```python
from build123d import *

# Parameters (mm, degrees)
SKETCH_1_R          = 40
EXTRUDE_1_DEPTH     = 11.8
SKETCH_2_R          = 2.15
SKETCH_2_R_2        = 1.75
CUT_EXTRUDE_1_DEPTH = 58.786157512
SKETCH_3_R          = 3.925
SKETCH_3_R_2        = 15.6
CUT_EXTRUDE_2_DEPTH = 58.786157512
SKETCH_5_R          = 2.9
SKETCH_5_R_2        = 3.5
CUT_EXTRUDE_4_DEPTH = 4
CHAMFER_1_SIZE      = 0.5


with BuildPart() as part:
    # 草图1 → 凸台-拉伸1 (new body)
    with BuildSketch(Plane.XY):
        Circle(SKETCH_1_R)
    extrude(amount=EXTRUDE_1_DEPTH)

    # 草图2 → 切除-拉伸1 (cut, through all)
    with BuildSketch(Plane(origin=(0, 0, 0), x_dir=(-1, 0, 0), z_dir=(0, 0, -1))):
        with Locations((-32.730643847, 10.1245665)):
            Circle(SKETCH_2_R)
        with Locations(Location((-32.730643847, -9.8754335, 0), (0, 0, 180))):
            Circle(SKETCH_2_R)
        with Locations((32.269356153, -9.8754335)):
            Circle(SKETCH_2_R)
        with Locations(Location((32.269356153, 10.1245665, 0), (0, 0, 180))):
            Circle(SKETCH_2_R)
        with Locations((-9.290643847, 33.9345665)):
            Circle(SKETCH_2_R_2)
        with Locations(Location((8.829356153, 33.9345665, 0), (0, 0, 180))):
            Circle(SKETCH_2_R_2)
        with Locations((8.829356153, -33.6854335)):
            Circle(SKETCH_2_R_2)
        with Locations(Location((-9.290643847, -33.6854335, 0), (0, 0, 180))):
            Circle(SKETCH_2_R_2)
    extrude(amount=-CUT_EXTRUDE_1_DEPTH, mode=Mode.SUBTRACT)

    # 草图3 → 切除-拉伸2 (cut, through all)
    with BuildSketch(Plane(origin=(0, 0, 0), x_dir=(-1, 0, 0), z_dir=(0, 0, -1))):
        with Locations((0, 31.5)):
            Circle(SKETCH_3_R)
        with Locations((27.279800219, 15.75)):
            Circle(SKETCH_3_R)
        with Locations((27.279800219, -15.75)):
            Circle(SKETCH_3_R)
        with Locations((0, -31.5)):
            Circle(SKETCH_3_R)
        with Locations((-27.279800219, -15.75)):
            Circle(SKETCH_3_R)
        with Locations((-27.279800219, 15.75)):
            Circle(SKETCH_3_R)
        Circle(SKETCH_3_R_2)
    extrude(amount=-CUT_EXTRUDE_2_DEPTH, mode=Mode.SUBTRACT)

    # 草图5 → 切除-拉伸4 (cut)
    with BuildSketch(Plane.XY.offset(11.8)):
        with Locations((-8.829356153, -33.6854335)):
            Circle(SKETCH_5_R)
        with Locations((-8.829356153, 33.9345665)):
            Circle(SKETCH_5_R)
        with Locations((-32.269356153, 10.1245665)):
            Circle(SKETCH_5_R_2)
        with Locations((-32.269356153, -9.8754335)):
            Circle(SKETCH_5_R_2)
        with Locations((9.290643847, 33.9345665)):
            Circle(SKETCH_5_R)
        with Locations((32.730643847, 10.1245665)):
            Circle(SKETCH_5_R_2)
        with Locations((32.730643847, -9.8754335)):
            Circle(SKETCH_5_R_2)
        with Locations((9.290643847, -33.6854335)):
            Circle(SKETCH_5_R)
    extrude(amount=-CUT_EXTRUDE_4_DEPTH, mode=Mode.SUBTRACT)

    # 倒角1
    # the kernel refuses this chamfer: 0.5 mm, written as the material it takes off along each edge
    with BuildSketch(Plane(origin=(0, 31.5, 11.8), x_dir=(-1, 0, 0), z_dir=(0, -1, 0))) as chamfer_1_piece_1:
        Polygon((3.925 + CHAMFER_1_SIZE, 0), (3.925, CHAMFER_1_SIZE), (3.925, 0), align=None)
    revolve(axis=Axis((0, 31.5, 11.8), (0, 0, -1)), mode=Mode.SUBTRACT)
    with BuildSketch(Plane(origin=(0, -31.5, 11.8), x_dir=(-1, 0, 0), z_dir=(0, -1, 0))) as chamfer_1_piece_2:
        Polygon((3.925 + CHAMFER_1_SIZE, 0), (3.925, CHAMFER_1_SIZE), (3.925, 0), align=None)
    revolve(axis=Axis((0, -31.5, 11.8), (0, 0, -1)), mode=Mode.SUBTRACT)
    with BuildSketch(Plane(origin=(-27.279800219, -15.75, 11.8), x_dir=(-1, 0, 0), z_dir=(0, -1, 0))) as chamfer_1_piece_3:
        Polygon((3.925 + CHAMFER_1_SIZE, 0), (3.925, CHAMFER_1_SIZE), (3.925, 0), align=None)
    revolve(axis=Axis((-27.279800219, -15.75, 11.8), (0, 0, -1)), mode=Mode.SUBTRACT)
    with BuildSketch(Plane(origin=(-27.279800219, 15.75, 11.8), x_dir=(-1, 0, 0), z_dir=(0, -1, 0))) as chamfer_1_piece_4:
        Polygon((3.925 + CHAMFER_1_SIZE, 0), (3.925, CHAMFER_1_SIZE), (3.925, 0), align=None)
    revolve(axis=Axis((-27.279800219, 15.75, 11.8), (0, 0, -1)), mode=Mode.SUBTRACT)
    with BuildSketch(Plane(origin=(27.279800219, -15.75, 11.8), x_dir=(-1, 0, 0), z_dir=(0, -1, 0))) as chamfer_1_piece_5:
        Polygon((3.925 + CHAMFER_1_SIZE, 0), (3.925, CHAMFER_1_SIZE), (3.925, 0), align=None)
    revolve(axis=Axis((27.279800219, -15.75, 11.8), (0, 0, -1)), mode=Mode.SUBTRACT)
    with BuildSketch(Plane(origin=(27.279800219, 15.75, 11.8), x_dir=(-1, 0, 0), z_dir=(0, -1, 0))) as chamfer_1_piece_6:
        Polygon((3.925 + CHAMFER_1_SIZE, 0), (3.925, CHAMFER_1_SIZE), (3.925, 0), align=None)
    revolve(axis=Axis((27.279800219, 15.75, 11.8), (0, 0, -1)), mode=Mode.SUBTRACT)


solid = part.part
```
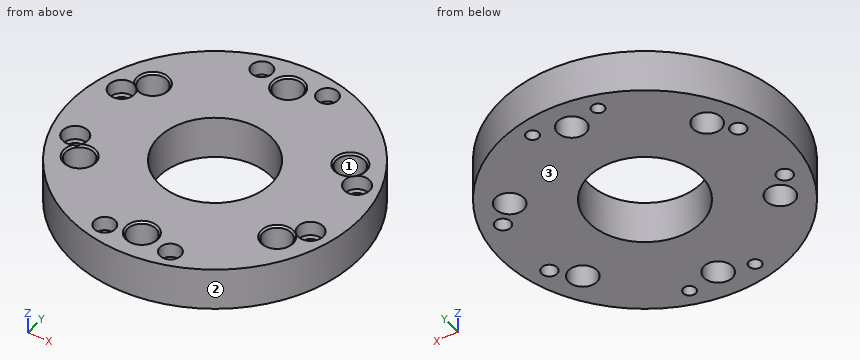
Work out the finished part from the listing and answer in its coordinate system (mm). Face numbers are marked on the shaded views. Give positions to 0.01 mm unless a question says otherwise; leave off trailing zeros. Loops run counter-clockwise (first coordinate to the right, second up) from the corner with the lowest first, then second, coordinate; pieces in that order, holes last. Notation, with made-up numbers: (0, 22) - (9, 22) arc R10 cw to (9, 41) - close; hole circle Ø3 at (-8.5, 73.5). An arc over 180 degrees is marked (long way). One line per question, with ' | ' between items.
(1) Each of these flat-tipped pins is pushed along its axis until it touches: pin 1 Ø1.5 at (y, z) = (8, 8.5) entering from -X; pin 2 Ø5 at (x, z) = (11.5, 2.5) entering from -Y; pin 3 Ø7 at (x, y) = (27.28, 15.75) entering from +Z; pin 4 Ø1.5 at (y, z) = (21.5, 9.5) entering from +X. Where does it stop, or does it pass through?
Recorded:
pin 1: stops at x = -39.34 | pin 2: stops at y = -38.97 | pin 3: passes through | pin 4: stops at x = 34.2
(2) The part is cut by section D-D (x = -13.5). Write down the section's boundary in (y, z), then the cut area to 3 significant figures.
Recorded:
outline: (-37.65, 0) - (-7.82, 0) - (-7.82, 11.8) - (-37.65, 11.8) - close; (7.82, 0) - (37.65, 0) - (37.65, 11.8) - (7.82, 11.8) - close | area: 704 mm²
(3) The part is cut by section C-C (z = 8.75). Count the separate pieces of the cut face and the enclosed holes in it, then the cut area to 3 significant figures.
Recorded:
separate pieces: 1 | enclosed holes: 15 | area: 3,710 mm²
(4) The part is cut by section B-B (x = 0). Write down the section's boundary in (y, z) (3 decimals), then the cut area to 3 significant figures.
Recorded:
outline: (-40, 0) - (-35.425, 0) - (-35.425, 11.3) - (-35.925, 11.8) - (-40, 11.8) - close; (-27.575, 0) - (-15.6, 0) - (-15.6, 11.8) - (-27.075, 11.8) - (-27.575, 11.3) - close; (15.6, 0) - (27.575, 0) - (27.575, 11.3) - (27.075, 11.8) - (15.6, 11.8) - close; (35.425, 0) - (40, 0) - (40, 11.8) - (35.925, 11.8) - (35.425, 11.3) - close | area: 390 mm²
(5) The mould has two halves that part along Y. Classify the marked faces 1, 2 and 3: +Y half, -Y half, draft (parallel to the pull), parting line (faces both ways), or undercut.
Recorded:
face 1: undercut | face 2: parting line | face 3: draft
(6) The part is cut by section A-A (y = 0). Write down the section's boundary in (x, z).
Recorded:
outline: (-40, 0) - (-15.6, 0) - (-15.6, 11.8) - (-40, 11.8) - close; (15.6, 0) - (40, 0) - (40, 11.8) - (15.6, 11.8) - close
(7) Straight lines are drawn through the part: probe 1 along X at (y, z) = (14, 7.5); probe 2 along Y at (x, z) = (1, 1.75); probe 3 along Y at (x, z) = (-26, 8.5). For each, find the intervals that lie inside material, in ascending order.
Recorded:
probe 1: x = -37.47 to -30.79, -23.77 to -6.88, 6.88 to 23.77, 30.79 to 37.47 | probe 2: y = -39.99 to -35.3, -27.7 to -15.57, 15.57 to 27.7, 35.3 to 39.99 | probe 3: y = -30.4 to -19.46, -12.04 to 12.04, 19.46 to 30.4
